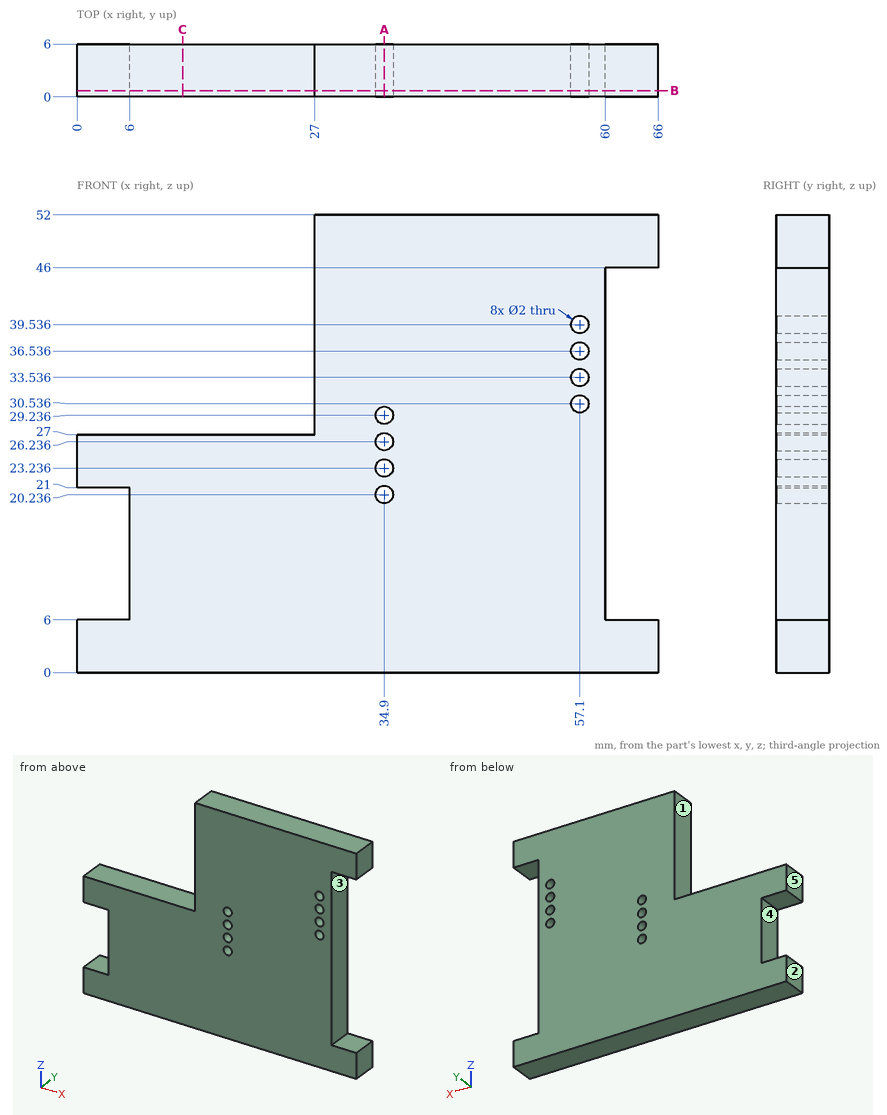
Study the drawing (mm; zero at the part's minimum x, y, z) and answer. A direction names the side the tool comes from. Give positions to 0.01 mm unless a question says otherwise; leave off trailing zeros. Write each loop counter-clockwise with the first axis right and the second up, starting at its lowest first coordinate (ties: lowest second). Pieces come first, ordered by that corner, then holes. Notation, with made-up numbers: M -12,59 L 29,59 A11 ccw 29,80 Z; hole C 15.25,46 d1. An arc over 180 degrees is marked long. Put each result on its own line as item: value. Start each with the question number.
1. This flat-tipped pin is pushed along its axis until it touches: pin 1 Ø1.8 at (y, z) = (4.5, 28) entering from +X. Where does it stop, or does it pass through?
2. The part is cut by section A-A, the plane x = 34.9. Give the vertices of the cut face in (y, z).
3. Consider line 1 along Z through (x, y) = (35, 4.9); line 2 along Z through (x, y) = (57.1, 4.75); line 3 along Z through (x, y) = (20, 1.2). Determine where each line is inside the solid, lowest interval first.
4. For a pull along Z with two mould halves and no side action, classify the marked faces 4 and 5 as released by +Z, released by -Z, zero draft, split by the parting line, or undercut.
5. The part is cut by section B-B, the plane y = 0.7. Give the number of separate pieces and of enclosed holes in the cut face, and give its area (3 significant figures).
6. Which of the six approach directions +Z, -Z, +X, -X, +Y, -Y give full straight-line access (tool end or side, diameter ignored) to the marked faces 1, 2 and 3?
7. The part is cut by section C-C, the plane x = 12. Give the vertices of the cut face in (y, z).
Final values:
1. pin 1: stops at x = 60
2. outline: M 0,0 L 6,0 L 6,19.24 L 0,19.24 Z; M 0,21.24 L 6,21.24 L 6,22.24 L 0,22.24 Z; M 0,24.24 L 6,24.24 L 6,25.24 L 0,25.24 Z; M 0,27.24 L 6,27.24 L 6,28.24 L 0,28.24 Z; M 0,30.24 L 6,30.24 L 6,52 L 0,52 Z
3. line 1: z = 0 to 19.24, 21.23 to 22.24, 24.23 to 25.24, 27.23 to 28.24, 30.23 to 52
3. line 2: z = 0 to 29.54, 31.54 to 32.54, 34.54 to 35.54, 37.54 to 38.54, 40.54 to 52
3. line 3: z = 0 to 27
4. face 4: undercut
4. face 5: zero draft
5. separate pieces: 1
5. enclosed holes: 8
5. area: 2,400 mm²
6. face 1: +Z, -X, +Y, -Y
6. face 2: +Z, -Z, -X, +Y, -Y
6. face 3: +X, +Y, -Y
7. outline: M 0,0 L 6,0 L 6,27 L 0,27 Z
